from build123d import *

# Parameters (mm, degrees)
F1_DEPTH = 3.175
F2_W     = 7.62
F2_H     = 50.8
F3_DEPTH = 12.7
F4_R     = 25.4
F5_R     = 5.08


with BuildPart() as f1:
    # F0 (on Front) → F1 (new body, symmetric)
    with BuildSketch(Plane.XZ):
        Polygon((123.498452, 101.6), (-123.498452, 101.6), (-119.0625, 0), (119.0625, 0), align=None)
    extrude(amount=F1_DEPTH, both=True)

    # F2 (on Front) → F3 (cut, symmetric)
    with BuildSketch(Plane.XZ):
        with Locations((-40.64, 76.2)):
            Rectangle(F2_W, F2_H)
        with Locations((40.64, 76.2)):
            Rectangle(F2_W, F2_H)
    extrude(amount=F3_DEPTH, both=True, mode=Mode.SUBTRACT)

    # F4
    f4_edges = [f1.edges().sort_by_distance(p)[0] for p in [
        (-119.0625, 0, 0),
        (119.0625, 0, 0),
    ]]
    fillet(f4_edges, radius=F4_R)

    # F5
    f5_edges = [f1.edges().sort_by_distance(p)[0] for p in [
        (-123.498452, 0, 101.6),
        (123.498452, 0, 101.6),
    ]]
    fillet(f5_edges, radius=F5_R)


solid = f1.part
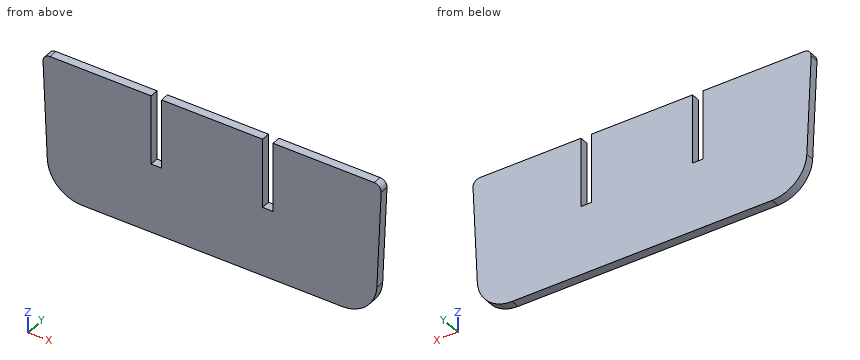
CAD build for the part. Positions are in the model's coordinates, mm. Coordinates: 2 decimals unless noted, no trailing zeros. Write each loop counter-clockwise with the first axis right and the second up, starting at its lowest first coordinate (ties: lowest second). Pieces come first, ordered by that corner, then holes. Notation, with made-up numbers: M 43.25,30.5 L 49.25,30.5 A13 ccw 49.25,37.5 Z; hole C -18.5,7 d11. An arc over 180 degrees is marked long. Answer as a JSON object with one key per item and string values. Group by question number.
1) Wall check: line 1 (X direction, y = 0.75, z = 67.5); line 2 (X direction, y = -0.25, z = 62); line 3 (Z direction, x = -41, y = 2). Give the ranges that are in metal, low to high. Write a range as from..to.
2) Saw through at B-B (y = 0.75). Write the cut outline in (x, z).
3) Saw through at C-C (z = 79). Write the cut outline in (x, y) (3 decimals), plus the area to 3 significant figures.
4) Saw through at D-D (z = 21.5). Write the cut outline in (x, y) (3 decimals), plus the area to 3 significant figures.
5) Saw through at A-A (z = 53). Write the cut outline in (x, y) (3 decimals).
6) Pin check, flat tips, straight feed: pin 1 Ø3 at (y, z) = (0, 66) entering from +X; pin 2 Ø1.9 at (y, z) = (0, 77) entering from -X; pin 3 Ø1.5 at (y, z) = (0, 33) entering from +X. Stop position of each tip, or through.
Values follow:
{
 "1": {"line 1": "x = -122.01..-44.45, -36.83..36.83, 44.45..122.01", "line 2": "x = -121.77..-44.45, -36.83..36.83, 44.45..121.77", "line 3": "z = 0..50.8"},
 "2": {"outline": "M -123.27,96.3 L -120.12,24.29 A25.4 ccw -94.75,0 L 94.75,0 A25.4 ccw 120.12,24.29 L 123.27,96.3 A5.08 ccw 118.19,101.6 L 44.45,101.6 L 44.45,50.8 L 36.83,50.8 L 36.83,101.6 L -36.83,101.6 L -36.83,50.8 L -44.45,50.8 L -44.45,101.6 L -118.19,101.6 A5.08 ccw Z"},
 "3": {"outline": "M -122.512,-3.175 L -44.45,-3.175 L -44.45,3.175 L -122.512,3.175 Z; M -36.83,-3.175 L 36.83,-3.175 L 36.83,3.175 L -36.83,3.175 Z; M 44.45,-3.175 L 122.512,-3.175 L 122.512,3.175 L 44.45,3.175 Z", "area": "1,460 mm2"},
 "4": {"outline": "M -119.846,-3.175 L 119.846,-3.175 L 119.846,3.175 L -119.846,3.175 Z", "area": "1,520 mm2"},
 "5": {"outline": "M -121.377,-3.175 L -44.45,-3.175 L -44.45,3.175 L -121.377,3.175 Z; M -36.83,-3.175 L 36.83,-3.175 L 36.83,3.175 L -36.83,3.175 Z; M 44.45,-3.175 L 121.377,-3.175 L 121.377,3.175 L 44.45,3.175 Z"},
 "6": {"pin 1": "stops at x = 122.01", "pin 2": "stops at x = -122.47", "pin 3": "stops at x = 120.54"}
}
